Geometry check sheet. Reference: the model listing, model coordinates, mm. Face numbers are marked on the shaded views. A direction names the side the tool comes from. Give positions to 0.01 mm unless a question says otherwise; leave off trailing zeros. Write each loop counter-clockwise with the first axis right and the second up, starting at its lowest first coordinate (ties: lowest second). Pieces come first, ordered by that corner, then holes. Notation, with made-up numbers: (86.5, 5) - (136.5, 5) arc R24 cw to (136.5, 33) - close; hole circle Ø1 at (66.5, 11). An arc over 180 degrees is marked (long way). Use a Markdown table: item, result.
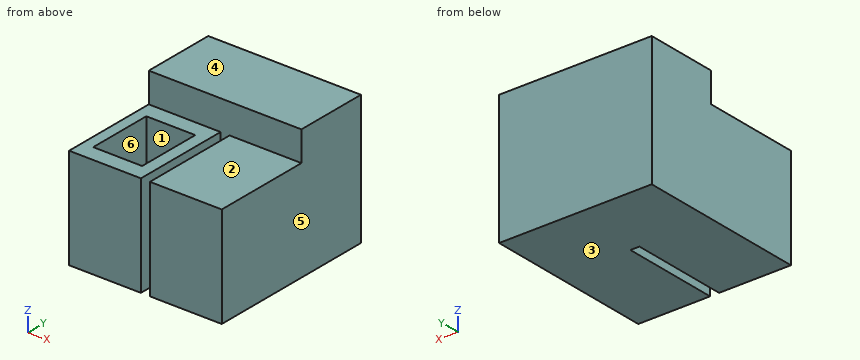
```python
from build123d import *

# Parameters (mm, degrees)
F0_W     = 25.4
F0_H     = 31.1311839489
F0_H_2   = 33.6493795661
F1_DEPTH = 101.6
F2_W     = 55.88
F2_H     = 78.4819734454
F3_DEPTH = 76.2
F4_W     = 38.1
F4_H     = 25.4
F5_DEPTH = 50.8


with BuildPart() as f1:
    # F0 (on Top) → F1 (new body)
    with BuildSketch(Plane.XY):
        Polygon((50.8, 38.1), (50.8, 0), (67.9685074601, 0), (67.9685074601, 38.1), (80.6685074601, 38.1), (106.0685074601, 38.1), (118.7685074601, 38.1), (118.7685074601, 56.9148101586), (0, 56.9148101586), (0, 38.1), (12.7, 38.1), (38.1, 38.1), align=None)
        Polygon((67.9685074601, 38.1), (67.9685074601, 0), (118.7685074601, 0), (118.7685074601, 38.1), (106.0685074601, 38.1), (106.0685074601, 4.4506204339), (80.6685074601, 4.4506204339), (80.6685074601, 38.1), align=None)
        Polygon((0, 38.1), (0, 0), (50.8, 0), (50.8, 38.1), (38.1, 38.1), (38.1, 6.9688160511), (12.7, 6.9688160511), (12.7, 38.1), align=None)
        with Locations((25.4, 22.5344080255)):
            Rectangle(F0_W, F0_H)
        with Locations((93.3685074601, 21.2753102169)):
            Rectangle(F0_W, F0_H_2)
    extrude(amount=-F1_DEPTH)

    # F2 (on face) → F3 (join)
    with BuildSketch(Plane.XZ):
        with Locations((27.94, -62.3590132773)):
            Rectangle(F2_W, F2_H)
        with Locations((90.8285074601, -62.3590132773)):
            Rectangle(F2_W, F2_H)
    extrude(amount=F3_DEPTH)

    # F4 (on face) → F5 (cut)
    with BuildSketch(Plane.XY.offset(-23.1180265546)):
        with Locations((27.4676065892, -25.4)):
            Rectangle(F4_W, F4_H)
        with Locations((27.4676065892, -50.8)):
            Rectangle(F4_W, F4_H)
    extrude(amount=-F5_DEPTH, mode=Mode.SUBTRACT)


solid = f1.part
```
1) Section check A-A on z = -62.5. Record the boundary of the cut face in (x, y).
Working result:
| item | result |
|---|---|
| outline | (0, -76.2) - (55.88, -76.2) - (55.88, 0) - (62.89, 0) - (62.89, -76.2) - (118.77, -76.2) - (118.77, 56.91) - (0, 56.91) - close; hole (8.42, -63.5) - (46.52, -63.5) - (46.52, -12.7) - (8.42, -12.7) - close |
2) Section check B-B on y = -23.5. Record the boundary of the cut face in (x, z), then the cut area to 3 significant figures.
Working result:
| item | result |
|---|---|
| outline | (0, -101.6) - (55.88, -101.6) - (55.88, -23.12) - (46.52, -23.12) - (46.52, -73.92) - (8.42, -73.92) - (8.42, -23.12) - (0, -23.12) - close; (62.89, -101.6) - (118.77, -101.6) - (118.77, -23.12) - (62.89, -23.12) - close |
| area | 6,840 mm² |
3) Section check D-D on x = 54. Record the boundary of the cut face in (y, z).
Working result:
| item | result |
|---|---|
| outline | (-76.2, -101.6) - (56.91, -101.6) - (56.91, 0) - (0, 0) - (0, -23.12) - (-76.2, -23.12) - close |
4) Set-up check for the marked faces 1, 2 and 3: record each of +Z, -Z, +X, -X, +Y, -Y from which the full face is reachable in a straight line by a thin tool's end or side.
Working result:
| item | result |
|---|---|
| face 1 | +Z |
| face 2 | +Z, +X, -X, -Y |
| face 3 | -Z, +X, -X, +Y, -Y |
5) Section check C-C on z = -87.5. Record the boundary of the cut face in (x, y).
Working result:
| item | result |
|---|---|
| outline | (0, -76.2) - (55.88, -76.2) - (55.88, 0) - (62.89, 0) - (62.89, -76.2) - (118.77, -76.2) - (118.77, 56.91) - (0, 56.91) - close |
6) Depth check by flat-ended pin: P1, Ø11.5, axis at x = 32.5, y = -29, coming from the +Z side. Enter the tip coordinate at first touch or a pass-through.
Working result:
| item | result |
|---|---|
| P1 | stops at z = -73.92 |
7) Material ranges on L1, parallel to X at y = -28, z = -47; L2, parallel to Y at x = 10, z = -51.5; L3, parallel to X at y = -67.5, z = -95, recorded low to high. Write a range as from..to.
Working result:
| item | result |
|---|---|
| L1 | x = 0..8.42, 46.52..55.88, 62.89..118.77 |
| L2 | y = -76.2..-63.5, -12.7..56.91 |
| L3 | x = 0..55.88, 62.89..118.77 |
8) Mould release check, pull along X, two halves, no side actions. Record for the marked faces 4, 5 and 6: pulls with the +X half, pulls with the -X half, needs draft (parallel to the pull), parting line crosses it, or undercut.
Working result:
| item | result |
|---|---|
| face 4 | needs draft |
| face 5 | pulls with the +X half |
| face 6 | undercut |
